Geometry check sheet. Reference: the model listing, model coordinates, mm. Face numbers are marked on the shaded views. A direction names the side the tool comes from. Round coordinates to 2 decimals unless told otherwise and drop trailing zeros. Loops run counter-clockwise (first coordinate to the right, second up) from the corner with the lowest first, then second, coordinate; pieces in that order, holes last.
```python
from build123d import *

# Parameters (mm, degrees)
SKETCH2_R               = 2.55
CUT_EXTRUDE1_DEPTH      = 36
SKETCH3_W               = 5.9
SKETCH3_H               = 2.6
CUT_EXTRUDE2_DEPTH      = 11
SKETCH4_R               = 4.5
SKETCH4_R_2             = 9
CUT_EXTRUDE3_DEPTH      = 11
CUT_EXTRUDE4_DEPTH      = 61
CUT_EXTRUDE4_DEPTH_BACK = 81
SKETCH5_R               = 1.682339559


with BuildPart() as part:
    # Sketch1 → Revolve2 (revolve)
    with BuildSketch(Plane(origin=(0, 0, 0), x_dir=(0, 0, -1), z_dir=(1, 0, 0)), mode=Mode.PRIVATE) as revolve2_sk:
        Polygon((0, 0), (0, 50), (-1, 50), (-1, 49), (-3, 49), (-3, 50), (-4, 50), (-4, 12), (-13.5, 12), (-13.5, 0), align=None)
    revolve(revolve2_sk.sketch.rotate(Axis((0, 0, 13.5), (0, 0, -1)), 90), axis=Axis((0, 0, 13.5), (0, 0, -1)))

    # Sketch2 → Cut-Extrude1 (cut)
    with BuildSketch(Plane.XY.offset(13.5)):
        Circle(SKETCH2_R)
    extrude(amount=-CUT_EXTRUDE1_DEPTH, mode=Mode.SUBTRACT)

    # Sketch3 → Cut-Extrude2 (cut)
    with BuildSketch(Plane.XY.offset(13.5)):
        with Locations((0, 6)):
            Rectangle(SKETCH3_W, SKETCH3_H)
        with Locations((0, -6)):
            Rectangle(SKETCH3_W, SKETCH3_H)
    extrude(amount=-CUT_EXTRUDE2_DEPTH, mode=Mode.SUBTRACT)

    # Sketch4 → Cut-Extrude3 (cut)
    with BuildSketch(Plane.XY.offset(4)):
        with Locations((0, 33.75)):
            Circle(SKETCH4_R)
        with Locations((0, -33.75)):
            Circle(SKETCH4_R)
        with Locations((33.75, 0)):
            Circle(SKETCH4_R)
        with Locations((-33.75, 0)):
            Circle(SKETCH4_R)
        with Locations((-17.995867581, 17.995867581)):
            Circle(SKETCH4_R_2)
        with Locations((17.995867581, 17.995867581)):
            Circle(SKETCH4_R_2)
        with Locations((17.995867581, -17.995867581)):
            Circle(SKETCH4_R_2)
        with Locations((-17.27525282, -18.688716917)):
            Circle(SKETCH4_R_2)
    extrude(amount=-CUT_EXTRUDE3_DEPTH, mode=Mode.SUBTRACT)

    # Sketch5 → Cut-Extrude4 (cut, two sides: drawn at the far end of the back side and taken through both)
    with BuildSketch(Plane(origin=(0, 4.7, 0), x_dir=(1, 0, 0), z_dir=(0, 1, 0)).offset(-CUT_EXTRUDE4_DEPTH_BACK)):
        with Locations(Location((0, -9.5, 0), (0, 0, 90))):
            Circle(SKETCH5_R)
    extrude(amount=CUT_EXTRUDE4_DEPTH + CUT_EXTRUDE4_DEPTH_BACK, mode=Mode.SUBTRACT)


solid = part.part
```
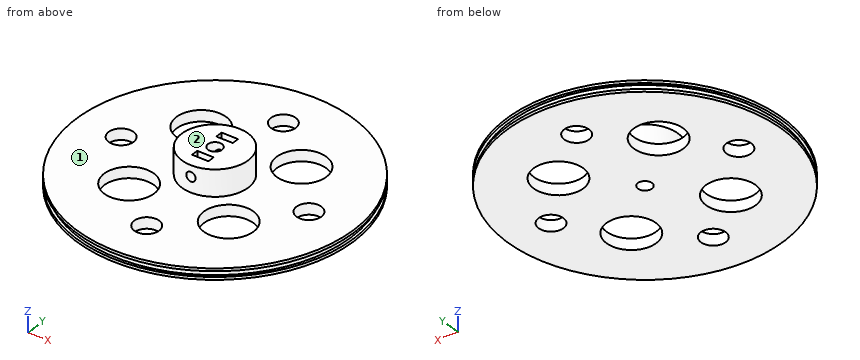
1) Sectioned sample at D-D, the plane x = 33.75. Record the cut outline in (y, z), then the cut area to 3 significant figures.
Report:
outline: (-36.89, 0) - (-4.5, 0) - (-4.5, 4) - (-36.89, 4) - (-36.89, 3) - (-35.52, 3) - (-35.52, 1) - (-36.89, 1) - close; (4.5, 0) - (36.89, 0) - (36.89, 1) - (35.52, 1) - (35.52, 3) - (36.89, 3) - (36.89, 4) - (4.5, 4) - close
area: 254 mm2
2) Sectioned sample at B-B, the plane y = -32. Record the cut outline in (x, z).
Report:
outline: (-38.42, 0) - (-4.15, 0) - (-4.15, 4) - (-38.42, 4) - (-38.42, 3) - (-37.11, 3) - (-37.11, 1) - (-38.42, 1) - close; (4.15, 0) - (38.42, 0) - (38.42, 1) - (37.11, 1) - (37.11, 3) - (38.42, 3) - (38.42, 4) - (4.15, 4) - close
3) Sectioned sample at C-C, the plane z = 9.5. Record the cut outline in (x, y).
Report:
outline: (-2.95, -7.3) - (-2.95, -4.7) - (-1.68, -4.7) - (-1.68, -1.92) arc R2.55 cw to (-1.68, 1.92) - (-1.68, 4.7) - (-2.95, 4.7) - (-2.95, 7.3) - (-1.68, 7.3) - (-1.68, 11.88) arc R12 ccw to (-1.68, -11.88) - (-1.68, -7.3) - close; (1.68, -11.88) arc R12 ccw to (1.68, 11.88) - (1.68, 7.3) - (2.95, 7.3) - (2.95, 4.7) - (1.68, 4.7) - (1.68, 1.92) arc R2.55 cw to (1.68, -1.92) - (1.68, -4.7) - (2.95, -4.7) - (2.95, -7.3) - (1.68, -7.3) - close
4) Access from +Z, -Z, +X, -X, +Y, -Y to the whole of each face (thin tool, end or side, straight path). Record for the marked faces 1 and 2.
Report:
face 1: +Z
face 2: +Z, +X, -X, +Y, -Y
5) Scan lines: line 1 along X through (y, z) = (15.5, 0.5); line 2 along X through (y, z) = (21.5, 1.5); line 3 along Z through (x, y) = (-7, -34). Record each from-to range of solid material in increasing order.
Report:
line 1: x = -47.54 to -26.64, -9.35 to 9.35, 26.64 to 47.54
line 2: x = -44.03 to -26.29, -9.71 to 9.71, 26.29 to 44.03
line 3: z = 0 to 4
6) Sectioned sample at A-A, the plane x = 0. State how many separate pieces and enclosed holes the cut face has, then the cut area to 3 significant figures.
Report:
separate pieces: 8
enclosed holes: 0
area: 380 mm2
7) Gauge pin test, flat ends, axial feed: pin 1 (16 mm diameter, centred on x = 18, y = -18, fed in from -Z); pin 2 (4.5 mm diameter, centred on x = -1, z = 6, fed in from +Y); pin 3 (2 mm diameter, centred on y = 11, z = 6, fed in from -X); pin 4 (12 mm diameter, centred on x = -31, y = -23, fed in from +Z). Record the tip position at first contact, or that the pin passes through.
Report:
pin 1: passes through
pin 2: stops at y = 50
pin 3: stops at x = -6.63
pin 4: stops at z = 4
